Part model, mm, in its own coordinate system. A direction names the side the tool comes from. Round coordinates to 2 decimals unless told otherwise and drop trailing zeros. Order: outer loops, then holes, each group sorted by start corner. A loop starts at its lowest first (then second) coordinate and runs counter-clockwise, first axis right, second up. Notation, with made-up numbers: (89.5, 9) -> (148.5, 9) arc R25 cw to (148.5, 22) -> close; hole circle Ø5 at (-34, 72). An arc over 180 degrees is marked (long way). Return JSON: item names as keys, results as strings. Group by question number.
Autodesk Inventor part; units mm, degrees
ref_plane "YZ Plane" through (0, 0, 0) normal (1, 0, 0) x (0, 1, 0)
ref_plane "XZ Plane" through (0, 0, 0) normal (0, 1, 0) x (-1, 0, 0)
ref_plane "XY Plane" through (0, 0, 0) normal (0, 0, 1) x (1, 0, 0)
sketch "Sketch1" plane through (0, 0, 0) normal (0, 1, 0) x (-1, 0, 0)
  circle A0 centre (0, 0) radius 77
  circle A1 centre (0, 0) radius 74.5
  dimension "d0" = 154
  dimension "d1" = 149
extrude "Extrusion1" add sketch "Sketch1" along normal blind 140
sketch "Sketch2" plane through (0, 0, 0) normal (1, 0, 0) x (0, 1, 0)
  circle A0 centre (75, 0) radius 32
  line L0 (0, -77) -> (0, 77)
  point P0 (0, 0)
  dimension "d4" = 64
  dimension "d5" = 75
extrude "Extrusion2" cut sketch "Sketch2" against normal through all
sketch "Sketch3" plane through (0, 0, 0) normal (0, 0, 1) x (1, 0, 0)
  circle A0 centre (0, 90) radius 22
  line L0 (77, 0) -> (-77, 0)
  point P0 (0, 0)
  dimension "d8" = 44
  dimension "d9" = 90
extrude "Extrusion3" cut sketch "Sketch3" along normal through all both and the other way through all
equation "\"d5\" = h_w"
equation "\"h_w\" = 75"
properties part number "chamber"
(1) Pin check, flat tips, straight feed: P1, Ø2, axis at y = 63, z = 9.5, coming from the -X side; P2, Ø3, axis at y = 63, z = 56.5, coming from the +X side; P3, Ø8, axis at x = -47.5, y = 72.5, coming from the +Z side. Stop position of each tip, or through.
(2) Tool access for faces 4 (the cylindrical face through (-72.115, 50.791, 20.926)), 5 (the flat face through (40.3, 140, 63.1)): list every direction of +Z, -Z, +X, -X, +Y, -Y with a clear straight run to the whole face (end or side of a thin tool).
(3) Saw through at B-B, the plane y = 90. List the corners of the cut face in (x, z), and give its area (3 significant figures).
(4) Saw through at C-C, the plane x = 0. List the corners of the cut face in (y, z), and give its area (3 significant figures).
(5) Saw through at A-A, the plane z = 0. List the corners of the cut face in (x, y), and give its area (3 significant figures).
(6) Probe L1, parallel to X at y = 8, z = 1.5; L2, parallel to X at y = 84.5, z = 39.5; L3, parallel to Z at x = 60.5, y = 63.5. List the from-to ranges inside material, lowest first. Write a range as [from, to].
(7) Mould opens along X. For faces 1 (the cylindrical face through (10.15, 109.52, 74.05)), 2 (the cylindrical face through (76.926, 69.02, -3.386)), 3 (the flat face through (40.3, 0, 63.1)) say: pulls with the +X half, pulls with the -X half, needs draft (parallel to the pull), parting line crosses it, or undercut.
(8) Saw through at D-D, the plane z = 67.5. List the corners of the cut face in (x, y), and give its area (3 significant figures).
Results are:
{
 "1": {"P1": "stops at x = 73.76", "P2": "stops at x = 53.89", "P3": "stops at z = 63.54"},
 "2": {"face 4": "-X", "face 5": "+Z, -Z, +X, -X, +Y"},
 "3": {"outline": "(-71.62, -28.27) arc R77 ccw to (-22, -73.79) -> (-22, -71.18) arc R74.5 cw to (-68.93, -28.27) -> close; (-71.62, 28.27) -> (-68.93, 28.27) arc R74.5 cw to (-22, 71.18) -> (-22, 73.79) arc R77 ccw to start; (22, -73.79) arc R77 ccw to (22, 73.79) -> (22, 71.18) arc R74.5 cw to (22, -71.18) -> close", "area": "822 mm^2"},
 "4": {"outline": "(0, -77) -> (68, -77) -> (68, -74.5) -> (0, -74.5) -> close; (0, 74.5) -> (68, 74.5) -> (68, 77) -> (0, 77) -> close; (112, -77) -> (140, -77) -> (140, -74.5) -> (112, -74.5) -> close; (112, 74.5) -> (140, 74.5) -> (140, 77) -> (112, 77) -> close", "area": "480 mm^2"},
 "5": {"outline": "(-77, 0) -> (-74.5, 0) -> (-74.5, 43) -> (-77, 43) -> close; (-77, 107) -> (-74.5, 107) -> (-74.5, 140) -> (-77, 140) -> close; (74.5, 0) -> (77, 0) -> (77, 140) -> (74.5, 140) -> close", "area": "540 mm^2"},
 "6": {"L1": "x = [-76.99, -74.48], [74.48, 76.99]", "L2": "x = [-66.1, -63.17], [63.17, 66.1]", "L3": "z = [-47.63, -43.47], [43.47, 47.63]"},
 "7": {"face 1": "undercut", "face 2": "parting line crosses it", "face 3": "needs draft"},
 "8": {"outline": "(-37.05, 0) -> (-31.53, 0) -> (-31.53, 140) -> (-37.05, 140) -> close; (31.53, 0) -> (37.05, 0) -> (37.05, 140) -> (31.53, 140) -> close", "area": "1,550 mm^2"}
}
